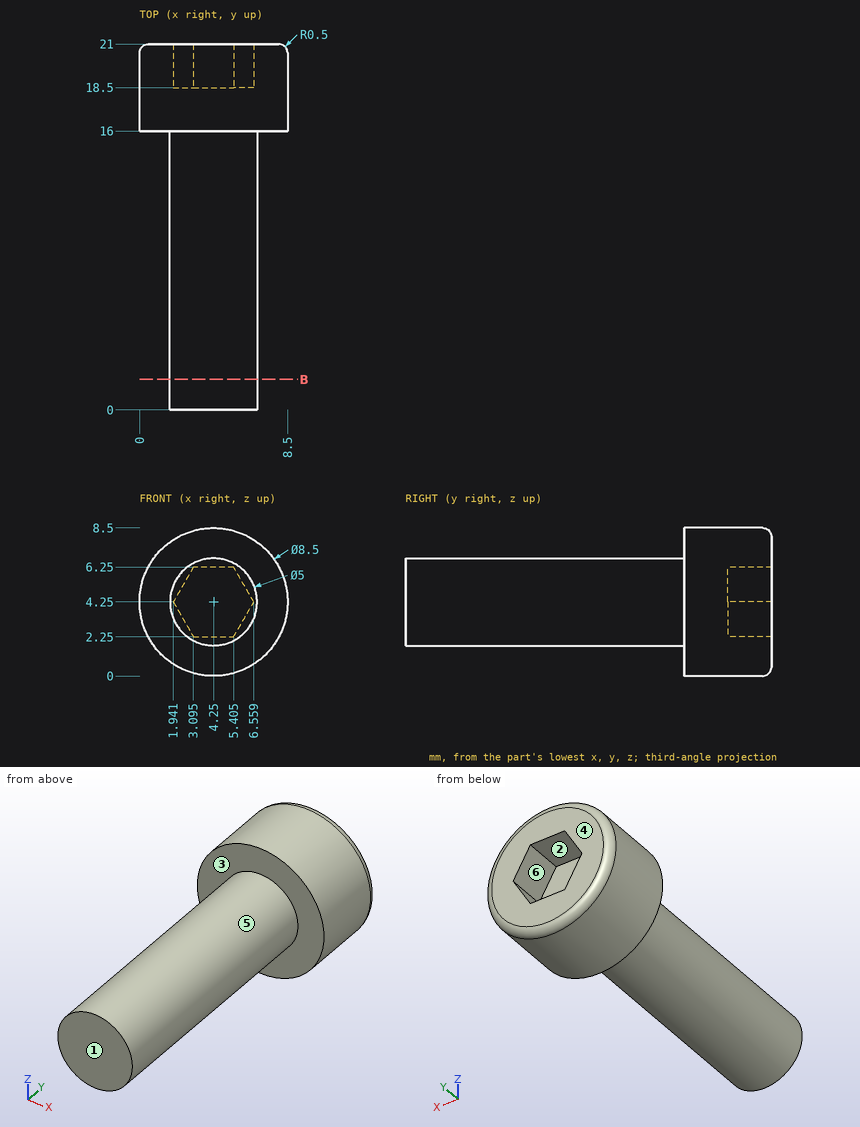
The drawing under review shows one solid part. Ordinate dimensions are in mm from its lowest x, y, z. A direction names the side the tool comes from. Round coordinates to 2 decimals unless told otherwise and drop trailing zeros. Loops run counter-clockwise (first coordinate to the right, second up) from the corner with the lowest first, then second, coordinate; pieces in that order, holes last. Notation, with made-up numbers: (71, -39.75) -> (109, -39.75) arc R36 ccw to (109, -4.75) -> close; hole circle Ø11 at (33.25, -26.5). An arc over 180 degrees is marked (long way). Answer in a Markdown table with one row per item.
1) Draft analysis for pull direction X (two halves, no side actions). For the marked faces 4, 5 and 6, state which applies: pulls with the +X half, pulls with the -X half, needs draft (parallel to the pull), parting line crosses it, or undercut.
Taken from the geometry:
| item | result |
|---|---|
| face 4 | needs draft |
| face 5 | parting line crosses it |
| face 6 | undercut |
2) Tool access review of the marked faces 1, 2 and 3: name each direction out of +Z, -Z, +X, -X, +Y, -Y from which nothing blocks a thin tool from reaching the whole face with its end or side.
Taken from the geometry:
| item | result |
|---|---|
| face 1 | +Z, -Z, +X, -X, -Y |
| face 2 | +Y |
| face 3 | -Y |
3) Wall thickness on line 1 along Y through (x, z) = (1, 2.75); line 2 along X through (y, z) = (17.5, 0.5); line 3 along Y through (x, z) = (3, 3.5): over which ranges is each line inside the solid? List them lowest first.
Taken from the geometry:
| item | result |
|---|---|
| line 1 | y = 16 to 21 |
| line 2 | x = 2.25 to 6.25 |
| line 3 | y = 0 to 18.5 |
4) For pin 1 Ø2 at (x, z) = (2.5, 4) entering from +Y; pin 2 Ø2 at (x, y) = (7, 4.5) entering from -Z (1 decimal); pin 3 Ø1 at (x, y) = (6.5, 2) entering from +Z (1 decimal); pin 4 Ø1 at (y, z) = (6.5, 7) entering from +X, all flat-tipped, find the tip position at first contact; note any pin that passes through.
Taken from the geometry:
| item | result |
|---|---|
| pin 1 | stops at y = 21 |
| pin 2 | stops at z = 2.5 |
| pin 3 | stops at z = 6 |
| pin 4 | stops at x = 5.34 |
5) Consider section B-B, the plane y = 1.75. Write out the cut boundary in (x, z).
Taken from the geometry:
| item | result |
|---|---|
| outline | circle Ø5 at (4.25, 4.25) |
